from build123d import *

# Parameters (mm, degrees)
SKETCH1_W                                       = 279.4
SKETCH1_H                                       = 241.3
BOSS_EXTRUDE1_DEPTH                             = 12.7
SKETCH2_R                                       = 34.1376
CUT_EXTRUDE1_DEPTH                              = 274.640060115
F_3_8_16_TAPPED_HOLE1_AT_2_COUNT                = 2
F_3_8_16_TAPPED_HOLE1_AT_2_PITCH                = 60.3504
F_3_8_16_TAPPED_HOLE1_AT_3_COUNT                = 2
F_3_8_16_TAPPED_HOLE1_AT_3_PITCH                = 184.783475994
F_3_8_16_TAPPED_HOLE1_AT_4_COUNT                = 2
F_3_8_16_TAPPED_HOLE1_AT_4_PITCH                = 174.6504
CSK_FOR_12_FLAT_HEAD_MACHINE_SCREW1_D           = 5.6134
CSK_FOR_12_FLAT_HEAD_MACHINE_SCREW1_CSINK_D     = 11.1252
CSK_FOR_12_FLAT_HEAD_MACHINE_SCREW1_CSINK_ANGLE = 82
CUT_EXTRUDE2_DEPTH                              = 7.9502
CUT_EXTRUDE3_DEPTH                              = 4.7752
CSK_FOR_8_FLAT_HEAD_MACHINE_SCREW1_D            = 4.3053
CSK_FOR_8_FLAT_HEAD_MACHINE_SCREW1_CSINK_D      = 8.4328
CSK_FOR_8_FLAT_HEAD_MACHINE_SCREW1_CSINK_ANGLE  = 82
CUT_EXTRUDE4_DEPTH                              = 274.640060115
FILLET1_R                                       = 3.175
CUT_EXTRUDE5_START                              = -6.35
CUT_EXTRUDE5_DEPTH                              = 6.35
FILLET2_R                                       = 3.175
CUT_EXTRUDE6_REACH                              = 278.815
CUT_EXTRUDE6_START                              = 3.175


# Read off the part's stored shape, not the designer's step: Cut-Extrude5
with BuildPart() as part:
    # Sketch1 → Boss-Extrude1 (new body)
    with BuildSketch(Plane.XY):
        with Locations((0, -114.3)):
            Rectangle(SKETCH1_W, SKETCH1_H)
    extrude(amount=BOSS_EXTRUDE1_DEPTH)

    # Sketch2 → Cut-Extrude1 (cut, through all)
    with BuildSketch(Plane.XY):
        with Locations((-57.15, -57.15)):
            Circle(SKETCH2_R)
        with Locations((57.15, -57.15)):
            Circle(SKETCH2_R)
    extrude(amount=CUT_EXTRUDE1_DEPTH, mode=Mode.SUBTRACT)

    # Sketch3 → 3/8-16 Tapped Hole1 (revolve, cut)
    with BuildSketch(Plane(origin=(87.3252, -26.9748, 0), x_dir=(0, 1, 0), z_dir=(1, 0, 0))):
        Polygon((0, 0), (0, 12.7), (5.08, 12.7), (3.96875, 11.58875), (3.96875, 1.11125), (5.08, 0), align=None)
    f_3_8_16_tapped_hole1 = revolve(axis=Axis((87.3252, -26.9748, -6.35), (0, 0, 1)), mode=Mode.SUBTRACT)

    # 3/8-16 Tapped Hole1 at 2: 3/8-16 Tapped Hole1 ×2
    with Locations(*[(0, -i * F_3_8_16_TAPPED_HOLE1_AT_2_PITCH, 0) for i in range(1, F_3_8_16_TAPPED_HOLE1_AT_2_COUNT)]):
        add(f_3_8_16_tapped_hole1, mode=Mode.SUBTRACT)

    # 3/8-16 Tapped Hole1 at 3: 3/8-16 Tapped Hole1 ×2
    with Locations(*[Vector(-0.9451624343615008, -0.3266006317688955, 0) * (i * F_3_8_16_TAPPED_HOLE1_AT_3_PITCH) for i in range(1, F_3_8_16_TAPPED_HOLE1_AT_3_COUNT)]):
        add(f_3_8_16_tapped_hole1, mode=Mode.SUBTRACT)

    # 3/8-16 Tapped Hole1 at 4: 3/8-16 Tapped Hole1 ×2
    with Locations(*[(-i * F_3_8_16_TAPPED_HOLE1_AT_4_PITCH, 0, 0) for i in range(1, F_3_8_16_TAPPED_HOLE1_AT_4_COUNT)]):
        add(f_3_8_16_tapped_hole1, mode=Mode.SUBTRACT)

    # CSK for #12 Flat Head Machine Screw1 (through all)
    with Locations(Plane(origin=(0, 0, 0), x_dir=(-1, 0, 0), z_dir=(0, 0, -1))):
        with Locations((42.9, -121.25), (7.9, -121.25), (7.9, -196.25), (42.9, -196.25)):
            CounterSinkHole(CSK_FOR_12_FLAT_HEAD_MACHINE_SCREW1_D / 2, CSK_FOR_12_FLAT_HEAD_MACHINE_SCREW1_CSINK_D / 2, counter_sink_angle=CSK_FOR_12_FLAT_HEAD_MACHINE_SCREW1_CSINK_ANGLE)

    # Sketch8 → Cut-Extrude2 (cut)
    with BuildSketch(Plane.XY.offset(12.7)):
        with BuildLine():
            Line((-113.538, -107.95), (-61.087, -107.95))
            ThreePointArc((-61.087, -107.95), (-56.058056572, -110.033056572), (-53.975, -115.062))
            Line((-53.975, -115.062), (-53.975, -208.788))
            ThreePointArc((-53.975, -208.788), (-56.058056572, -213.816943428), (-61.087, -215.9))
            Line((-61.087, -215.9), (-113.538, -215.9))
            ThreePointArc((-113.538, -215.9), (-118.566943428, -213.816943428), (-120.65, -208.788))
            Line((-120.65, -208.788), (-120.65, -115.062))
            ThreePointArc((-120.65, -115.062), (-118.566943428, -110.033056572), (-113.538, -107.95))
        make_face()
        with BuildLine():
            Line((10.287, -107.95), (113.538, -107.95))
            ThreePointArc((113.538, -107.95), (118.566943428, -110.033056572), (120.65, -115.062))
            Line((120.65, -115.062), (120.65, -208.788))
            ThreePointArc((120.65, -208.788), (118.566943428, -213.816943428), (113.538, -215.9))
            Line((113.538, -215.9), (10.287, -215.9))
            ThreePointArc((10.287, -215.9), (5.258056572, -213.816943428), (3.175, -208.788))
            Line((3.175, -208.788), (3.175, -115.062))
            ThreePointArc((3.175, -115.062), (5.258056572, -110.033056572), (10.287, -107.95))
        make_face()
        with BuildLine():
            Line((-26.2255, -107.95), (-24.5745, -107.95))
            ThreePointArc((-24.5745, -107.95), (-19.545556572, -110.033056572), (-17.4625, -115.062))
            Line((-17.4625, -115.062), (-17.4625, -208.788))
            ThreePointArc((-17.4625, -208.788), (-19.545556572, -213.816943428), (-24.5745, -215.9))
            Line((-24.5745, -215.9), (-26.2255, -215.9))
            ThreePointArc((-26.2255, -215.9), (-31.254443428, -213.816943428), (-33.3375, -208.788))
            Line((-33.3375, -208.788), (-33.3375, -115.062))
            ThreePointArc((-33.3375, -115.062), (-31.254443428, -110.033056572), (-26.2255, -107.95))
        make_face()
    extrude(amount=-CUT_EXTRUDE2_DEPTH, mode=Mode.SUBTRACT)

    # Sketch9 → Cut-Extrude3 (cut)
    with BuildSketch(Plane.XY.offset(12.7)):
        with BuildLine():
            Line((-103.0351, 0.635), (103.0351, 0.635))
            ThreePointArc((103.0351, 0.635), (109.204535955, -1.920464045), (111.76, -8.0899))
            Line((111.76, -8.0899), (111.76, -93.5101))
            ThreePointArc((111.76, -93.5101), (109.204535955, -99.679535955), (103.0351, -102.235))
            Line((103.0351, -102.235), (-103.0351, -102.235))
            ThreePointArc((-103.0351, -102.235), (-109.204535955, -99.679535955), (-111.76, -93.5101))
            Line((-111.76, -93.5101), (-111.76, -8.0899))
            ThreePointArc((-111.76, -8.0899), (-109.204535955, -1.920464045), (-103.0351, 0.635))
        make_face()
        with BuildLine():
            Line((108.077, -8.0899), (108.077, -93.5101))
            ThreePointArc((108.077, -93.5101), (106.60026168, -97.07526168), (103.0351, -98.552))
            Line((103.0351, -98.552), (-103.0351, -98.552))
            ThreePointArc((-103.0351, -98.552), (-106.60026168, -97.07526168), (-108.077, -93.5101))
            Line((-108.077, -93.5101), (-108.077, -8.0899))
            ThreePointArc((-108.077, -8.0899), (-106.60026168, -4.52473832), (-103.0351, -3.048))
            Line((-103.0351, -3.048), (103.0351, -3.048))
            ThreePointArc((103.0351, -3.048), (106.60026168, -4.52473832), (108.077, -8.0899))
        make_face(mode=Mode.SUBTRACT)
    extrude(amount=-CUT_EXTRUDE3_DEPTH, mode=Mode.SUBTRACT)

    # CSK for #8 Flat Head Machine Screw1 (through all)
    with Locations(Plane(origin=(0, 0, 0), x_dir=(-1, 0, 0), z_dir=(0, 0, -1))):
        with Locations((100.0252, -50.8), (0, -11.0998), (-100.0252, -50.8), (0, -90.4748)):
            CounterSinkHole(CSK_FOR_8_FLAT_HEAD_MACHINE_SCREW1_D / 2, CSK_FOR_8_FLAT_HEAD_MACHINE_SCREW1_CSINK_D / 2, counter_sink_angle=CSK_FOR_8_FLAT_HEAD_MACHINE_SCREW1_CSINK_ANGLE)

    # Sketch12 → Cut-Extrude4 (cut, through all)
    with BuildSketch(Plane.XY):
        with BuildLine():
            Line((-137.3378, 23.951822796), (-137.3378, -11.1252))
            ThreePointArc((-137.3378, -11.1252), (-139.42829606, -16.17210394), (-144.4752, -18.2626))
            Line((-144.4752, -18.2626), (-144.4752, 23.951822796))
            Line((-144.4752, 23.951822796), (-137.3378, 23.951822796))
        make_face()
    extrude(amount=CUT_EXTRUDE4_DEPTH, mode=Mode.SUBTRACT)

    # Fillet1
    fillet1_edges = [part.edges().sort_by_distance(p)[0] for p in [
        (-137.3378, 6.35, 6.35),
        (139.7, 6.35, 6.35),
        (139.7, -234.95, 6.35),
        (-139.7, -234.95, 6.35),
    ]]
    fillet(fillet1_edges, radius=FILLET1_R)

    # Cut-Extrude5 outline → Cut-Extrude5 (cut)
    with BuildSketch(Plane.XY.offset(12.7).offset(CUT_EXTRUDE5_START)):
        with BuildLine():
            Line((-133.35, -228.6), (-133.35, 6.35))
            Line((-133.35, 6.35), (-134.1628, 6.35))
            ThreePointArc((-134.1628, 6.35), (-136.40786403, 5.42006403), (-137.3378, 3.175))
            Line((-137.3378, 3.175), (-137.3378, -11.1252))
            ThreePointArc((-137.3378, -11.1252), (-137.955039295, -14.028643325), (-139.7, -16.429909579))
            Line((-139.7, -16.429909579), (-139.7, -231.775))
            ThreePointArc((-139.7, -231.775), (-138.77006403, -234.02006403), (-136.525, -234.95))
            Line((-136.525, -234.95), (136.525, -234.95))
            ThreePointArc((136.525, -234.95), (138.77006403, -234.02006403), (139.7, -231.775))
            Line((139.7, -231.775), (139.7, 3.175))
            ThreePointArc((139.7, 3.175), (138.77006403, 5.42006403), (136.525, 6.35))
            Line((136.525, 6.35), (133.35, 6.35))
            Line((133.35, 6.35), (133.35, -228.6))
            Line((133.35, -228.6), (-133.35, -228.6))
        make_face()
    extrude(amount=CUT_EXTRUDE5_DEPTH, mode=Mode.SUBTRACT)

    # Fillet2
    fillet2_edges = [part.edges().sort_by_distance(p)[0] for p in [
        (133.35, 6.35, 9.525),
        (-133.35, 6.35, 9.525),
        (133.35, -228.6, 9.525),
        (-133.35, -228.6, 9.525),
    ]]
    fillet(fillet2_edges, radius=FILLET2_R)

    # Sketch14 → Cut-Extrude6 (cut, up to next)
    with BuildSketch(Plane.XY.offset(CUT_EXTRUDE6_START), mode=Mode.PRIVATE) as cut_extrude6_sk1:
        with BuildLine():
            Line((144.5006, -12.7254), (162.7632, -12.7254))
            Line((162.7632, -12.7254), (162.7632, -33.3502))
            Line((162.7632, -33.3502), (144.5006, -33.3502))
            ThreePointArc((144.5006, -33.3502), (139.45369606, -31.25970394), (137.3632, -26.2128))
            Line((137.3632, -26.2128), (137.3632, -19.8628))
            ThreePointArc((137.3632, -19.8628), (139.45369606, -14.81589606), (144.5006, -12.7254))
        make_face()
    cut_extrude6_tool1 = extrude(cut_extrude6_sk1.sketch, amount=CUT_EXTRUDE6_REACH, mode=Mode.PRIVATE) & part.part
    # Sketch14 → Cut-Extrude6 (cut, up to next)
    with BuildSketch(Plane.XY.offset(CUT_EXTRUDE6_START), mode=Mode.PRIVATE) as cut_extrude6_sk2:
        with BuildLine():
            Line((144.5006, -195.2498), (162.7632, -195.2498))
            Line((162.7632, -195.2498), (162.7632, -215.8746))
            Line((162.7632, -215.8746), (144.5006, -215.8746))
            ThreePointArc((144.5006, -215.8746), (139.45369606, -213.78410394), (137.3632, -208.7372))
            Line((137.3632, -208.7372), (137.3632, -202.3872))
            ThreePointArc((137.3632, -202.3872), (139.45369606, -197.34029606), (144.5006, -195.2498))
        make_face()
    cut_extrude6_tool2 = extrude(cut_extrude6_sk2.sketch, amount=CUT_EXTRUDE6_REACH, mode=Mode.PRIVATE) & part.part
    add(cut_extrude6_tool1.solids().sort_by_distance((150.546907, -23.0378, 3.175))[0], mode=Mode.SUBTRACT)
    add(cut_extrude6_tool2.solids().sort_by_distance((150.546907, -205.5622, 3.175))[0], mode=Mode.SUBTRACT)


solid = part.part
Geometry: final body of the model. Coordinates: model frame, mm. A direction names the side the tool comes from. Give positions to 0.01 mm unless a question says otherwise; leave off trailing zeros. Loops run counter-clockwise (first coordinate to the right, second up) from the corner with the lowest first, then second, coordinate; pieces in that order, holes last. Notation, with made-up numbers: (-14.5, 40) - (0.5, 40) arc R27 ccw to (0.5, 58) - close; hole circle Ø6 at (33.5, 42.5). An arc over 180 degrees is marked (long way). One line per question, with ' | ' between items. Start each with the question number.
(1) Ray query, line 1 (Y direction, x = -114, z = 10.5); line 2 (Y direction, x = 57.15, z = 3.5); line 3 (Y direction, x = -7.9, z = 8.75) (3 decimals). Return the intervals inside material, ascending. Write a range as from..to.
(2) Section query C-C on y = -70. Return loops of the section in (x, z), then the cut area to 3 significant figures.
(3) Reachability of faces 1 (the flat face through (-17.462, -161, 9)), 2 (the conical face through (-41.543, -123.859, 3.016)) from +Z, -Z, +X, -X, +Y, -Y: full face, straight path, thin tool, end or side. Return the list, or none.
(4) Pull-direction query (Y, two-part tool) for faces 3 (the cylindrical face through (-31.31, -110.09, 8.78)), 4 (the flat face through (-2, -234.95, 3)), 5 (the flat face through (-139.7, -126, 3)), 6 (the cylindrical face through (109.272, -99.611, 10.346)); classes: released by +Y, released by -Y, zero draft, split by the parting line, or undercut.
(5) Contact query for flat-ended pins moving along their axis: pin 1 (2.5 mm diameter, centred on y = -153.5, z = 8.5, fed in from -X); pin 2 (1.4 mm diameter, centred on x = 47.5, z = 10.5, fed in from -Y); pin 3 (8 mm diameter, centred on x = -27.5, y = -172, fed in from +Z). Output: stop coordinate, or through.
(6) Section query B-B on x = 57.15. Return loops of the section in (y, z) (3 decimals).
The answers:
1) line 1: -228.6..-215.88, -107.97..6.35 | line 2: -234.95..-91.29, -23.01..6.35 | line 3: -228.6..-199.057, -193.443..-124.057, -118.443..-102.235, -98.552..-3.048, 0.635..6.35
2) outline: (-139.7, 0) - (-88.78, 0) - (-88.78, 12.7) - (-108.08, 12.7) - (-108.08, 7.92) - (-111.76, 7.92) - (-111.76, 12.7) - (-133.35, 12.7) - (-133.35, 6.35) - (-139.7, 6.35) - close; (-25.52, 0) - (25.52, 0) - (25.52, 12.7) - (-25.52, 12.7) - close; (88.78, 0) - (139.7, 0) - (139.7, 6.35) - (133.35, 6.35) - (133.35, 12.7) - (111.76, 12.7) - (111.76, 7.92) - (108.08, 7.92) - (108.08, 12.7) - (88.78, 12.7) - close | area: 1,830 mm2
3) face 1: +Z | face 2: -Z
4) face 3: undercut | face 4: released by -Y | face 5: zero draft | face 6: undercut
5) pin 1: x = -133.35 | pin 2: y = -228.6 | pin 3: z = 4.75
6) outline: (-234.95, 0) - (-91.288, 0) - (-91.288, 12.7) - (-98.552, 12.7) - (-98.552, 7.925) - (-102.235, 7.925) - (-102.235, 12.7) - (-107.95, 12.7) - (-107.95, 4.75) - (-215.9, 4.75) - (-215.9, 12.7) - (-228.6, 12.7) - (-228.6, 6.35) - (-234.95, 6.35) - close; (-23.012, 0) - (6.35, 0) - (6.35, 12.7) - (0.635, 12.7) - (0.635, 7.925) - (-3.048, 7.925) - (-3.048, 12.7) - (-23.012, 12.7) - close
